For this review, take the finished solid that the model builds, in its own axes (mm). A direction names the side the tool comes from. Give positions to 0.01 mm unless a question says otherwise; leave off trailing zeros. Order: outer loops, then holes, each group sorted by start corner. A loop starts at its lowest first (then second) coordinate and runs counter-clockwise, first axis right, second up. Notation, with made-up numbers: (75, 63) -> (126, 63) arc R38 cw to (126, 101) -> close; hole circle Ø6 at (-26.75, -6). An arc over 180 degrees is marked (long way). Return JSON: item names as keys, results as strings. Group by question number.
1) Insertion check: P1, Ø6, axis at x = 5, y = 4, coming from the +Z side. The pin has a flat end and moves straight along its axis. Give the tip position at first contact, or say it passes through.
2) For faces 5 (the face through (6, -2, -261)), 6 (the face through (6, -36, 261)), 7 (the face through (7, 108, 213)), 8 (the face through (6, -105, 249)), 9 (the face through (6, 60, 249)), list the 3-axis set-ups (+Z, -Z, +X, -X, +Y, -Y) from which the entire face can be reached by the end or side of a thin tool; tool diameter is ignored.
3) To check wall thickness, follow line 1 along Z through (x, y) = (5.5, -106); line 2 along Z through (x, y) = (5.5, -74.5); line 3 along Z through (x, y) = (0.5, 95.5). State the ranges of each line that lie inside material, in increasing order.
4) Add section A-A (x = 9.5). Give the boundary of the cut face in (y, z).
5) Add section B-B (y = -105). Give the boundary of the cut face in (x, z).
6) The part is to be moulded in two halves that separate along Z. For faces 1 (the face through (6, -75, 255)), 2 (the face through (6, 36, 261)), 3 (the face through (12, -2, 4)), 4 (the face through (6, 45, 255)), say which applies: released by +Z, released by -Z, zero draft, split by the parting line, or undercut.
from build123d import *

# Parameters (mm, degrees)
F1_DEPTH = 12
F3_DEPTH = 12
F5_DEPTH = 12


with BuildPart() as f1:
    # F0 (on Right) → F1 (new body)
    with BuildSketch(Plane.YZ):
        Polygon((120, 225), (120, 249), (96, 249), (90, 249), (78, 249), (72, 249), (48, 249), (42, 249), (30, 249), (24, 249), (-24, 249), (-30, 249), (-42, 249), (-48, 249), (-72, 249), (-78, 249), (-90, 249), (-96, 249), (-120, 249), (-120, -261), (120, -261), (120, 153), (108, 153), (108, 177), (120, 177), (120, 201), (108, 201), (108, 225), align=None)
        Polygon((-78, 249), (-72, 261), (-96, 261), (-90, 249), align=None)
        Polygon((-30, 249), (-24, 261), (-48, 261), (-42, 249), align=None)
        Polygon((42, 249), (48, 261), (24, 261), (30, 249), align=None)
        Polygon((90, 249), (96, 261), (72, 261), (78, 249), align=None)
    extrude(amount=F1_DEPTH)

    # F2 (on face) → F3 (join)
    with BuildSketch(Plane(origin=(0, 108, 0), x_dir=(-1, 0, 0), z_dir=(0, 1, 0))):
        Polygon((0, 219), (0, 225), (-12, 225), align=None)
        Polygon((0, 207), (-12, 201), (0, 201), align=None)
    extrude(amount=F3_DEPTH)

    # F4 (on face) → F5 (join)
    with BuildSketch(Plane(origin=(0, 108, 0), x_dir=(-1, 0, 0), z_dir=(0, 1, 0))):
        Polygon((0, 177), (-12, 177), (0, 171), align=None)
        Polygon((0, 159), (-12, 153), (0, 153), align=None)
    extrude(amount=F5_DEPTH)


solid = f1.part
Evaluation:
{
 "1": {"P1": "z = 249"},
 "2": {"face 5": "-Z, +X, -X, +Y, -Y", "face 6": "+Z, +X, -X, +Y, -Y", "face 7": "+X, +Y", "face 8": "+X, -X, -Y", "face 9": "+X, -X"},
 "3": {"line 1": "-261 to 249", "line 2": "-261 to 249, 256 to 261", "line 3": "-261 to 249, 260 to 261"},
 "4": {"outline": "(-120, -261) -> (120, -261) -> (120, 154.25) -> (108, 154.25) -> (108, 175.75) -> (120, 175.75) -> (120, 202.25) -> (108, 202.25) -> (108, 223.75) -> (120, 223.75) -> (120, 249) -> (90, 249) -> (96, 261) -> (72, 261) -> (78, 249) -> (42, 249) -> (48, 261) -> (24, 261) -> (30, 249) -> (-30, 249) -> (-24, 261) -> (-48, 261) -> (-42, 249) -> (-78, 249) -> (-72, 261) -> (-96, 261) -> (-90, 249) -> (-120, 249) -> close"},
 "5": {"outline": "(0, -261) -> (12, -261) -> (12, 249) -> (0, 249) -> close"},
 "6": {"face 1": "undercut", "face 2": "released by +Z", "face 3": "zero draft", "face 4": "undercut"}
}
